The figure shows three views and two pictorial views of one solid part (mm, origin at its lowest corner). Answer the questions. Coordinates: 2 decimals unless noted, no trailing zeros. Loops run counter-clockwise (first coordinate to the right, second up) from the corner with the lowest first, then second, coordinate; pieces in that order, holes last. Notation, with made-up numbers: M -7,11 L 8,11 A14 ccw 8,37 Z; hole C 66.25,-7 d6. An arc over 180 degrees is marked long. Answer as a JSON object with one key per item and string values. Group by question number.
1. Straight lines are drawn through the part: L1, parallel to Y at x = 24, z = 13; L2, parallel to X at y = 20, z = 31; L3, parallel to X at y = 25.5, z = 25.5. For each, find the intervals that lie inside material, in ascending order.
2. A cutting plane is placed at C-C on z = 8. Give the vertices of the cut face in (x, y).
3. A cutting plane is placed at A-A on y = 24. Give the vertices of the cut face in (x, z).
4. Determine the mould class of the marked faces 1, 2, 3 and 4 for opening direction X: released by +X, released by -X, zero draft, split by the parting line, or undercut.
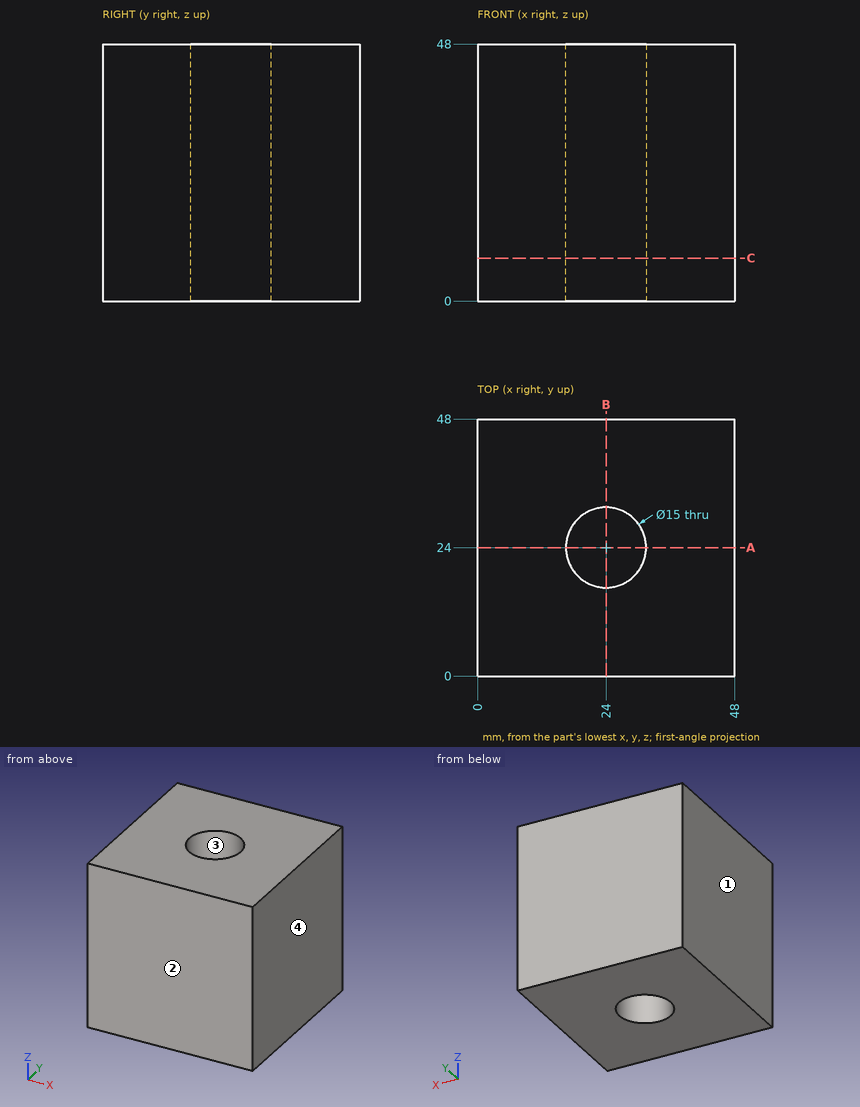
From the geometry:
{
 "1": {"L1": "y = 0 to 16.5, 31.5 to 48", "L2": "x = 0 to 17.66, 30.34 to 48", "L3": "x = 0 to 16.65, 31.35 to 48"},
 "2": {"outline": "M 0,0 L 48,0 L 48,48 L 0,48 Z; hole C 24,24 d15"},
 "3": {"outline": "M 0,0 L 16.5,0 L 16.5,48 L 0,48 Z; M 31.5,0 L 48,0 L 48,48 L 31.5,48 Z"},
 "4": {"face 1": "released by -X", "face 2": "zero draft", "face 3": "undercut", "face 4": "released by +X"}
}
